```python
from build123d import *

# Parameters (mm, degrees)
SKETCH1_W            = 32.9
SKETCH1_H            = 36
BOSS_EXTRUDE1_DEPTH  = 6.92
M8_CLEARANCE_HOLE1_D = 8.4
CHAMFER1_SIZE        = 0.508


with BuildPart() as part:
    # Sketch1 → Boss-Extrude1 (new body)
    with BuildSketch(Plane.XY):
        Rectangle(SKETCH1_W, SKETCH1_H)
    extrude(amount=BOSS_EXTRUDE1_DEPTH)

    # M8 Clearance Hole1 (through all)
    with Locations(Plane.XY.offset(6.92)):
        with Locations((-7.449999987, -9), (-7.449999987, 9)):
            Hole(M8_CLEARANCE_HOLE1_D / 2)

    # Chamfer1
    chamfer1_edges = [part.edges().sort_by_distance(p)[0] for p in [
        (-16.45, -18, 3.46),
    ]]
    chamfer(chamfer1_edges, length=CHAMFER1_SIZE)


solid = part.part
```
Read the model definition and answer for the solid it produces. Units are mm, in the model's axes. Coordinates: 2 decimals unless noted, no trailing zeros. Write each loop counter-clockwise with the first axis right and the second up, starting at its lowest first coordinate (ties: lowest second). Pieces come first, ordered by that corner, then holes. Notation, with made-up numbers: (-25.75, -15.75) -> (-3.75, -15.75) arc R19 ccw to (-3.75, 15.25) -> close; hole circle Ø11 at (87, 76.5). An arc over 180 degrees is marked (long way). Return JSON: item names as keys, results as strings.
1. A cutting plane is placed at B-B (z = 4.75). Determine the outline of the cut face in (x, y).
Found:
{"outline": "(-16.45, -17.49) -> (-15.94, -18) -> (16.45, -18) -> (16.45, 18) -> (-16.45, 18) -> close; hole circle Ø8.4 at (-7.45, -9); hole circle Ø8.4 at (-7.45, 9)"}
2. A cutting plane is placed at D-D (y = -11). Determine the outline of the cut face in (x, z).
Found:
{"outline": "(-16.45, 0) -> (-11.14, 0) -> (-11.14, 6.92) -> (-16.45, 6.92) -> close; (-3.76, 0) -> (16.45, 0) -> (16.45, 6.92) -> (-3.76, 6.92) -> close"}
3. Find the intervals of material crossed by line 1 along Y through (x, z) = (-7.45, 3); line 2 along Y through (x, z) = (-8.5, 2); line 3 along X through (y, z) = (-7, 2.75), in increasing order. Write a range as from..to.
Found:
{"line 1": "-18..-13.2, -4.8..4.8, 13.2..18", "line 2": "-18..-13.07, -4.93..4.93, 13.07..18", "line 3": "-16.45..-11.14, -3.76..16.45"}
4. Determine the mould class of faces 1 (the face through (16.45, 0, 3)), 2 (the face through (-6.54, -13.1, 3.41)), 3 (the face through (0, -18, 3)) for opening direction Y: pulls with the +Y half, pulls with the -Y half, needs draft (parallel to the pull), parting line crosses it, or undercut.
Found:
{"face 1": "needs draft", "face 2": "undercut", "face 3": "pulls with the -Y half"}
5. A cutting plane is placed at A-A (y = 9). Determine the outline of the cut face in (x, z), and give its area (3 significant figures).
Found:
{"outline": "(-16.45, 0) -> (-11.65, 0) -> (-11.65, 6.92) -> (-16.45, 6.92) -> close; (-3.25, 0) -> (16.45, 0) -> (16.45, 6.92) -> (-3.25, 6.92) -> close", "area": "170 mm2"}
6. A cutting plane is placed at C-C (x = -7.45). Determine the outline of the cut face in (y, z).
Found:
{"outline": "(-18, 0) -> (-13.2, 0) -> (-13.2, 6.92) -> (-18, 6.92) -> close; (-4.8, 0) -> (4.8, 0) -> (4.8, 6.92) -> (-4.8, 6.92) -> close; (13.2, 0) -> (18, 0) -> (18, 6.92) -> (13.2, 6.92) -> close"}
